Could you check a few things on this drawing? It's one solid part, dimensions in mm from its lowest x, y, z. Give positions to 0.01 mm unless a question says otherwise; leave off trailing zeros. Order: outer loops, then holes, each group sorted by start corner. A loop starts at its lowest first (then second) coordinate and runs counter-clockwise, first axis right, second up. Notation, with made-up numbers: (-19, -25.5) - (5, -25.5) arc R11 cw to (5, -7.5) - close; hole circle Ø4 at (62.5, -16.75). An arc over 180 degrees is marked (long way). Return JSON: item names as keys, results as strings.
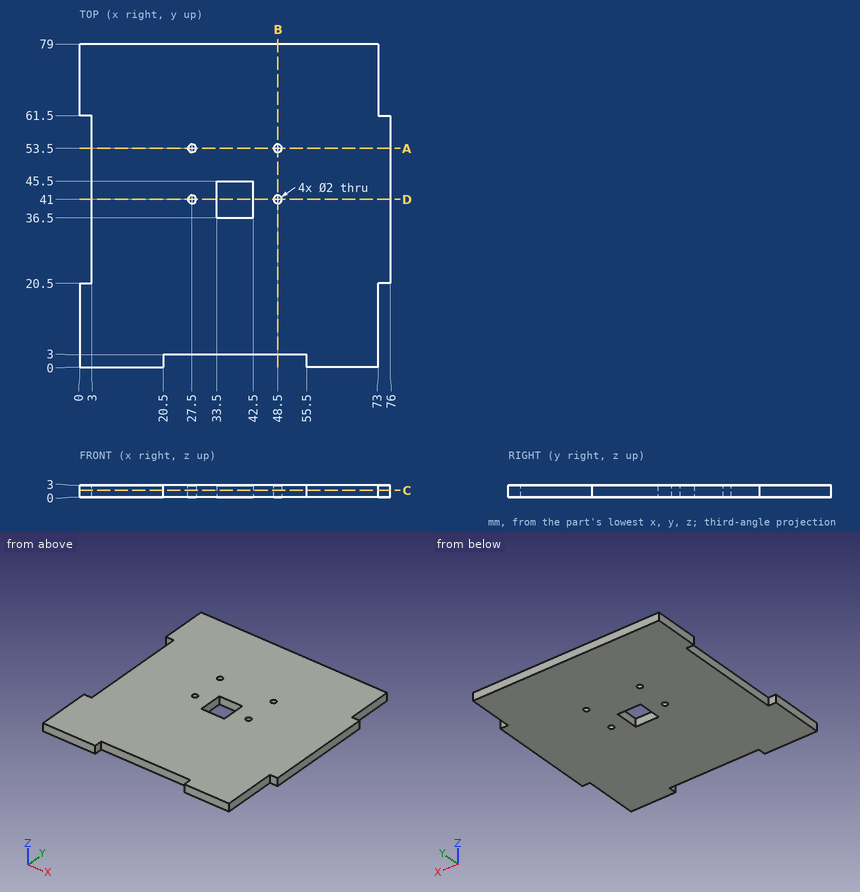
1. Suppose I cut it at D-D (y = 41). List the corners of the cut face in (x, z) for me.
Checks:
{"outline": "(3, 0) - (26.5, 0) - (26.5, 3) - (3, 3) - close; (28.5, 0) - (33.5, 0) - (33.5, 3) - (28.5, 3) - close; (42.5, 0) - (47.5, 0) - (47.5, 3) - (42.5, 3) - close; (49.5, 0) - (76, 0) - (76, 3) - (49.5, 3) - close"}
2. For pin 1 Ø0.9 at (y, z) = (34.5, 1.5) entering from -X, with a flat end and sliding along its axis, tell me the tip position at first contact or that it passes through.
Checks:
{"pin 1": "x = 3"}
3. Suppose I cut it at A-A (y = 53.5). List the corners of the cut face in (x, z) for me.
Checks:
{"outline": "(3, 0) - (26.5, 0) - (26.5, 3) - (3, 3) - close; (28.5, 0) - (47.5, 0) - (47.5, 3) - (28.5, 3) - close; (49.5, 0) - (76, 0) - (76, 3) - (49.5, 3) - close"}
4. Suppose I cut it at C-C (z = 1.7). List the corners of the cut face in (x, y) for me, plus the area to 3 significant figures.
Checks:
{"outline": "(0, 0) - (20.5, 0) - (20.5, 3) - (55.5, 3) - (55.5, 0) - (73, 0) - (73, 20.5) - (76, 20.5) - (76, 61.5) - (73, 61.5) - (73, 79) - (0, 79) - (0, 61.5) - (3, 61.5) - (3, 20.5) - (0, 20.5) - close; hole circle Ø2 at (27.5, 41); hole circle Ø2 at (27.5, 53.5); hole (33.5, 36.5) - (42.5, 36.5) - (42.5, 45.5) - (33.5, 45.5) - close; hole circle Ø2 at (48.5, 41); hole circle Ø2 at (48.5, 53.5)", "area": "5,570 mm^2"}
5. If I drill on L1, parallel to Y at x = 48.5, z = 2.3; L2, parallel to X at y = 37.5, z = 2.65; L3, parallel to Y at x = 22.5, z = 1.8, over which ranges is the centre line in solid material (lowest first)? Write a range as [from, to].
Checks:
{"L1": "[3, 40], [42, 52.5], [54.5, 79]", "L2": "[3, 33.5], [42.5, 76]", "L3": "[3, 79]"}
6. Suppose I cut it at B-B (x = 48.5). List the corners of the cut face in (y, z) for me, plus the area to 3 significant figures.
Checks:
{"outline": "(3, 0) - (40, 0) - (40, 3) - (3, 3) - close; (42, 0) - (52.5, 0) - (52.5, 3) - (42, 3) - close; (54.5, 0) - (79, 0) - (79, 3) - (54.5, 3) - close", "area": "216 mm^2"}
